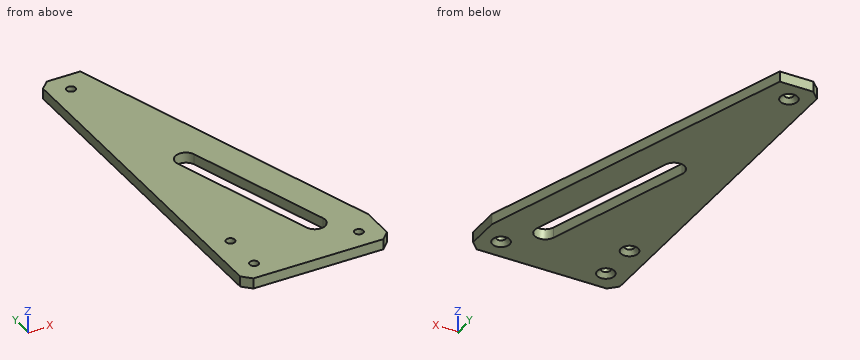
from build123d import *

# Parameters (mm, degrees)
SKETCH_1_R          = 2.1
EXTRUDE_1_DEPTH     = 2.5
CHAMFER_1_SIZE      = 4
CHAMFER_2_SIZE      = 2
CUT_EXTRUDE_1_DEPTH = 95.372930441


with BuildPart() as part:
    # 草图1 → 凸台-拉伸1 (new, symmetric)
    with BuildSketch(Plane.XY):
        Polygon((-35, 87.5), (-35, -87.5), (35, -87.5), (35, -67.5), (-15, 87.5), align=None)
        with Locations((-25, -77.5)):
            Circle(SKETCH_1_R, mode=Mode.SUBTRACT)
        with Locations((25, -77.5)):
            Circle(SKETCH_1_R, mode=Mode.SUBTRACT)
        with Locations((-25, 77.5)):
            Circle(SKETCH_1_R, mode=Mode.SUBTRACT)
        with Locations((-25, -57.5)):
            Circle(SKETCH_1_R, mode=Mode.SUBTRACT)
    extrude(amount=EXTRUDE_1_DEPTH, both=True)

    # 倒角1
    chamfer_1_edges = [part.edges().sort_by_distance(p)[0] for p in [
        (-35, -87.5, 0),
        (-35, 87.5, 0),
        (35, -87.5, 0),
    ]]
    chamfer(chamfer_1_edges, length=CHAMFER_1_SIZE)

    # 倒角2
    chamfer_2_edges = [part.edges().sort_by_distance(p)[0] for p in [
        (22.9, -77.5, -2.5),
        (-27.1, -77.5, -2.5),
        (-27.1, 77.5, -2.5),
        (-27.1, -57.5, -2.5),
    ]]
    chamfer(chamfer_2_edges, length=CHAMFER_2_SIZE)

    # 草图2 → 切除-拉伸1 (cut, through all)
    with BuildSketch(Plane(origin=(0, 0, -2.5), x_dir=(-1, 0, 0), z_dir=(0, 0, -1))):
        with BuildLine():
            Line((-17.130804412, -60.9649861), (5.241456911, 8.389024))
            ThreePointArc((5.241456911, 8.389024), (11.5350139, 11.612553189), (14.758543089, 5.318996201))
            Line((14.758543089, 5.318996201), (-7.613718234, -64.0350139))
            ThreePointArc((-7.613718234, -64.0350139), (-13.907275222, -67.258543089), (-17.130804412, -60.9649861))
        make_face()
    extrude(amount=-CUT_EXTRUDE_1_DEPTH, mode=Mode.SUBTRACT)


solid = part.part
Work out the finished part from the listing and answer in its coordinate system (mm). Round coordinates to 2 decimals unless told otherwise and drop trailing zeros. Write each loop counter-clockwise with the first axis right and the second up, starting at its lowest first coordinate (ties: lowest second). Pieces come first, ordered by that corner, then holes. Notation, with made-up numbers: (24, -15.75) - (65, -15.75) arc R19 cw to (65, 2.25) - close; hole circle Ø10 at (23.25, 26.5). An arc over 180 degrees is marked (long way). Answer in a Markdown table with one row per item. Add a question column.
1. Find the intervals of material crossed by line 1 along Y through (x, z) = (-25, 0.25); line 2 along X through (y, z) = (4.5, -0.5); line 3 along X through (y, z) = (-22, -0.35), in increasing order. Write a range as from..to.
2. Given pin 1 (1 mm diameter, centred on y = -41.5, z = 0.5, fed in from +X), flat-ended and moving along its own axis, determine where the tip first touches the part or whether it passes through.
3. A cutting plane is placed at A-A, the plane z = 0.7. Determine the outline of the cut face in (x, y).
4. A cutting plane is placed at B-B, the plane x = 11. Determine the outline of the cut face in (y, z), and give its area (3 significant figures).
5. A cutting plane is placed at D-D, the plane y = 77.5. Determine the outline of the cut face in (x, z), and give its area (3 significant figures).
6. A cutting plane is placed at C-C, the plane y = -35.5. Determine the outline of the cut face in (x, z), and give its area (3 significant figures).
Worked out:
| question | item | result |
|---|---|---|
| 1 | line 1 | -87.5..-79.6, -75.4..-59.6, -55.4..75.4, 79.6..87.5 |
| 1 | line 2 | -35..-14.49, -3.99..11.77 |
| 1 | line 3 | -35..-5.95, 4.56..20.32 |
| 2 | pin 1 | x = 26.77 |
| 3 | outline | (-35, -83.5) - (-31, -87.5) - (31, -87.5) - (35, -83.5) - (35, -67.5) - (-15, 87.5) - (-31, 87.5) - (-35, 83.5) - close; hole circle Ø4.2 at (-25, -77.5); hole circle Ø4.2 at (-25, -57.5); hole circle Ø4.2 at (-25, 77.5); hole (-14.76, 5.32) - (7.61, -64.04) arc R5 ccw to (17.13, -60.96) - (-5.24, 8.39) arc R5 ccw to start; hole circle Ø4.2 at (25, -77.5) |
| 4 | outline | (-87.5, -2.5) - (-67.31, -2.5) - (-67.31, 2.5) - (-87.5, 2.5) - close; (-41.96, -2.5) - (6.9, -2.5) - (6.9, 2.5) - (-41.96, 2.5) - close |
| 4 | area | 345 mm^2 |
| 5 | outline | (-35, -2.5) - (-29.1, -2.5) - (-27.1, -0.5) - (-27.1, 2.5) - (-35, 2.5) - close; (-22.9, -0.5) - (-20.9, -2.5) - (-11.77, -2.5) - (-11.77, 2.5) - (-22.9, 2.5) - close |
| 5 | area | 91.1 mm^2 |
| 6 | outline | (-35, -2.5) - (-1.59, -2.5) - (-1.59, 2.5) - (-35, 2.5) - close; (8.92, -2.5) - (24.68, -2.5) - (24.68, 2.5) - (8.92, 2.5) - close |
| 6 | area | 246 mm^2 |
